Here's the drawing with two shaded views (mm, measured from the low corner). I have some questions. Coordinates: 2 decimals unless noted, no trailing zeros. Order: outer loops, then holes, each group sorted by start corner. A loop starts at its lowest first (then second) coordinate and runs counter-clockwise, first axis right, second up. Notation, with made-up numbers: (47, 10) -> (94, 10) arc R29 cw to (94, 34) -> close; hole circle Ø2 at (10, 68.5). An arc over 180 degrees is marked (long way). Answer as a JSON object with one key per item and string values. Group by question number.
(1) I want a section at A-A, the plane y = 3. List the corners of the cut face in (x, z) for me, plus the area to 3 significant figures.
(2) For pin 1 (6 mm diameter, centred on x = 35, z = 74.5, fed in from +Y); pin 2 (0.9 mm diameter, centred on x = 31.5, y = 3.5, fed in from +Z); pin 3 (1.8 mm diameter, centred on y = 3.5, z = 4.5, fed in from -X), each with a flat end and sliding along its axis, tell me the tip position at first contact or that it passes through.
(3) If we mould it in two halves opening along Y, with no side actions, what happens to the marked faces 1, 2 and 3? For each: pulls with the +Y half, pulls with the -Y half, needs draft (parallel to the pull), parting line crosses it, or undercut.
(4) I want a section at D-D, the plane z = 93. List the corners of the cut face in (x, y) for me, plus the area to 3 significant figures.
(5) I want a section at C-C, the plane x = 57. List the corners of the cut face in (y, z) for me, plus the area to 3 significant figures.
(6) I want a section at B-B, the plane z = 3. List the corners of the cut face in (x, y) for me, plus the area to 3 significant figures.
(7) I need wall thicknesses on line 1 (Z direction, x = 46.5, y = 3); line 2 (Y direction, x = 45.75, z = 3); line 3 (Z direction, x = 60.95, y = 3). Which ranges of each line are inside material? Lowest first, please.
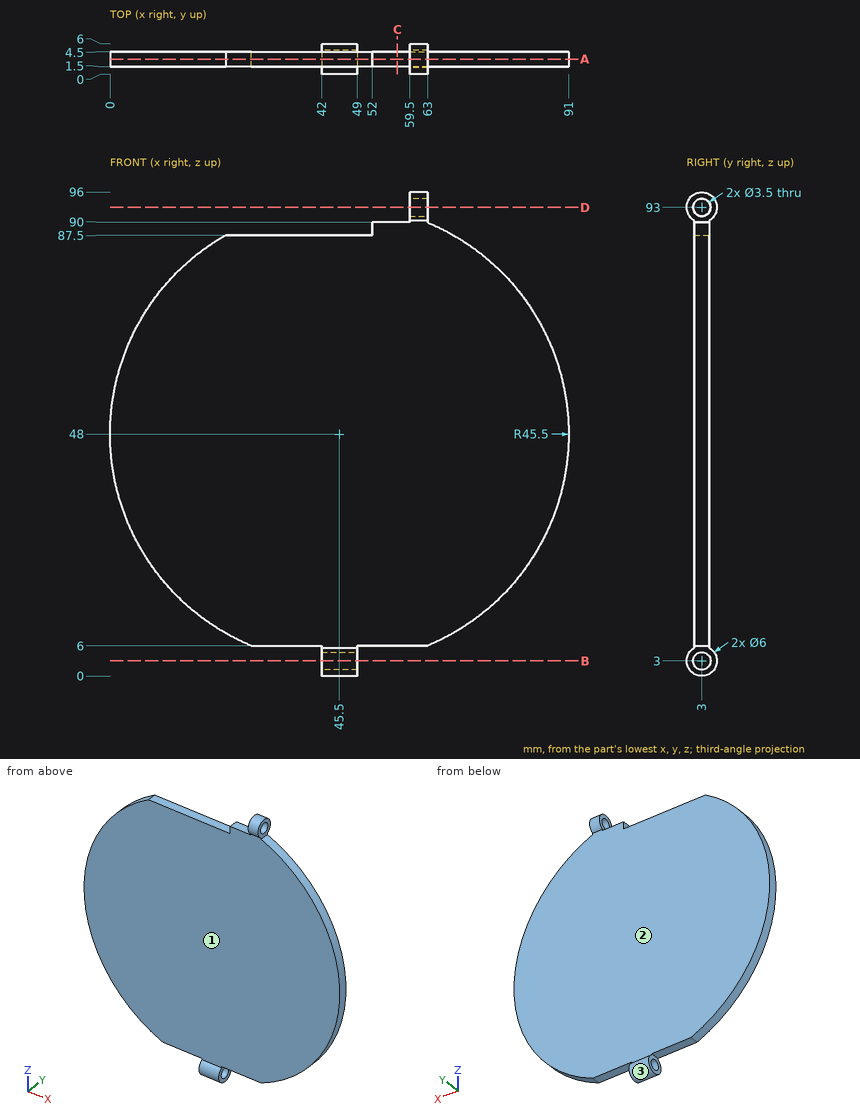
Computed values:
{
 "1": {"outline": "(22.92, 87.5) arc R45.5 ccw to (28, 6) -> (42, 6) -> (42, 4.75) -> (49, 4.75) -> (49, 6) -> (63, 6) arc R45.5 ccw to (63, 90) -> (63, 91.25) -> (59.5, 91.25) -> (59.5, 90) -> (52, 90) -> (52, 87.5) -> close; (42, 0) -> (49, 0) -> (49, 1.25) -> (42, 1.25) -> close; (59.5, 94.75) -> (63, 94.75) -> (63, 96) -> (59.5, 96) -> close", "area": "6,300 mm2"},
 "2": {"pin 1": "stops at y = 4.5", "pin 2": "stops at z = 87.5", "pin 3": "stops at x = 42"},
 "3": {"face 1": "pulls with the -Y half", "face 2": "pulls with the +Y half", "face 3": "parting line crosses it"},
 "4": {"outline": "(59.5, 0) -> (63, 0) -> (63, 1.25) -> (59.5, 1.25) -> close; (59.5, 4.75) -> (63, 4.75) -> (63, 6) -> (59.5, 6) -> close", "area": "8.75 mm2"},
 "5": {"outline": "(1.5, 6) -> (4.5, 6) -> (4.5, 90) -> (1.5, 90) -> close", "area": "252 mm2"},
 "6": {"outline": "(42, 0) -> (49, 0) -> (49, 1.25) -> (42, 1.25) -> close; (42, 4.75) -> (49, 4.75) -> (49, 6) -> (42, 6) -> close", "area": "17.5 mm2"},
 "7": {"line 1": "z = 0 to 1.25, 4.75 to 87.5", "line 2": "y = 0 to 1.25, 4.75 to 6", "line 3": "z = 6 to 91.25, 94.75 to 96"}
}
